```python
from build123d import *

# Parameters (mm, degrees)
F1_DEPTH      = 0.3175
F3_DEPTH      = 0.3185
F3_DEPTH_BACK = 0.3185


with BuildPart() as f1:
    # F0 (on Front) → F1 (new body, symmetric)
    with BuildSketch(Plane.XZ):
        Polygon((15.875, 0), (-15.875, 0), (-30.95, -18.9), (30.95, -18.9), align=None)
    extrude(amount=F1_DEPTH, both=True)

    # F2 (on Front) → F3 (cut, two sides)
    with BuildSketch(Plane.XZ) as f3_sk:
        with BuildLine():
            Line((-1.525, 0), (-4.825, 0))
            Line((-4.825, 0), (-4.825, -2.35))
            ThreePointArc((-4.825, -2.35), (-3.175, -4), (-1.525, -2.35))
            Line((-1.525, -2.35), (-1.525, 0))
        make_face()
        with BuildLine():
            Line((4.825, -2.35), (4.825, 0))
            Line((4.825, 0), (1.525, 0))
            Line((1.525, 0), (1.525, -2.35))
            ThreePointArc((1.525, -2.35), (3.175, -4), (4.825, -2.35))
        make_face()
    extrude(amount=-F3_DEPTH, mode=Mode.SUBTRACT)
    extrude(f3_sk.sketch, amount=F3_DEPTH_BACK, mode=Mode.SUBTRACT)


solid = f1.part
```
Could you check a few things on this model? Use its own coordinates, in mm. Round coordinates to 2 decimals unless told otherwise and drop trailing zeros. Order: outer loops, then holes, each group sorted by start corner. A loop starts at its lowest first (then second) coordinate and runs counter-clockwise, first axis right, second up. Notation, with made-up numbers: (41, -31) -> (70, -31) arc R9 ccw to (70, -24) -> close; hole circle Ø6 at (84, -9). An arc over 180 degrees is marked (long way). One line per question, with ' | ' between items.
Q1. If I drill on line 1 (X direction, y = 0.05, z = -1) (3 decimals); line 2 (X direction, y = 0.1, z = -0.75) (3 decimals); line 3 (Z direction, x = 17.5, y = -0.1), over which ranges is the centre line in solid material (lowest first)? Write a range as from..to.
Computed values:
line 1: -16.673..-4.825, -1.525..1.525, 4.825..16.673 | line 2: -16.473..-4.825, -1.525..1.525, 4.825..16.473 | line 3: -18.9..-2.04
Q2. If we section it at C-C on z = -12.25: Write out the boundary of the cut face in (x, y).
Computed values:
outline: (-25.65, -0.32) -> (25.65, -0.32) -> (25.65, 0.32) -> (-25.65, 0.32) -> close
Q3. If we section it at B-B on x = -22: Write out the boundary of the cut face in (y, z).
Computed values:
outline: (-0.32, -18.9) -> (0.32, -18.9) -> (0.32, -7.68) -> (-0.32, -7.68) -> close
Q4. We'd pull the mould along X, two halves only. Please class faces 1 (the face through (0, -0.318, -11)), 2 (the face through (23.518, -0.004, -9.582)), 3 (the face through (-3.2, 0, -4)): released by +X, released by -X, zero draft, split by the parting line, or undercut.
Computed values:
face 1: zero draft | face 2: released by +X | face 3: undercut
Q5. If we section it at A-A on y = 0.2: Write out the boundary of the cut face in (x, z) (3 decimals), plus the area to 3 significant figures.
Computed values:
outline: (-30.95, -18.9) -> (30.95, -18.9) -> (15.875, 0) -> (4.825, 0) -> (4.825, -2.35) arc R1.65 cw to (1.525, -2.35) -> (1.525, 0) -> (-1.525, 0) -> (-1.525, -2.35) arc R1.65 cw to (-4.825, -2.35) -> (-4.825, 0) -> (-15.875, 0) -> close | area: 861 mm²
